```python
from build123d import *

# Parameters (mm, degrees)
BOSS_EXTRUDE1_DEPTH = 6
FILLET1_R           = 6
FILLET2_R           = 4
BOSS_EXTRUDE2_DEPTH = 12
LPATTERN1_COUNT     = 6
LPATTERN1_PITCH     = 6
CUT_EXTRUDE1_DEPTH  = 26
SKETCH5_R           = 1.5
CUT_EXTRUDE4_DEPTH  = 124.180869367
SKETCH6_R           = 1.75
BOSS_EXTRUDE3_DEPTH = 3
SKETCH7_R           = 1.25
CUT_EXTRUDE6_DEPTH  = 1
SKETCH8_R           = 1.25
CUT_EXTRUDE7_DEPTH  = 1
CUT_EXTRUDE8_DEPTH  = 1


with BuildPart() as part:
    # Sketch1 → Boss-Extrude1 (new, symmetric)
    with BuildSketch(Plane(origin=(0, 0, 0), x_dir=(1, 0, 0), z_dir=(0, 1, 0))):
        with BuildLine():
            ThreePointArc((13.432245527, -50.487906924), (21.509028276, -53.088979862), (18.907955338, -61.165762611))
            Line((18.907955338, -61.165762611), (11, -67.286566673))
            Line((11, -67.286566673), (11, -117.286566673))
            Line((11, -117.286566673), (0, -117.286566673))
            Line((0, -117.286566673), (0, -110.286566673))
            Line((0, -110.286566673), (-20.129396013, -88.042299634))
            Line((-20.129396013, -88.042299634), (-31.928362438, -82.58479184))
            Line((-31.928362438, -82.58479184), (-27.730279519, -73.508663821))
            Line((-27.730279519, -73.508663821), (-24.896421124, -73.027946621))
            Line((-24.896421124, -73.027946621), (-12.941547125, -71))
            Line((-12.941547125, -71), (-4.10711559, -69.126148868))
            Line((-4.10711559, -69.126148868), (13.432245527, -50.487906924))
        make_face()
        Polygon((-12.941547125, -71), (-24.896421124, -73.027946621), (-36.603518956, -4.013862114), (-12.941547125, 0), align=None)
    extrude(amount=BOSS_EXTRUDE1_DEPTH, both=True)

    # Fillet1
    fillet1_edges = [part.edges().sort_by_distance(p)[0] for p in [
        (-36.603518956, 0, 4.013862114),
        (-12.941547125, 0, 0),
    ]]
    fillet(fillet1_edges, radius=FILLET1_R)

    # Fillet2
    fillet2_edges = [part.edges().sort_by_distance(p)[0] for p in [
        (0, 0, 117.286566673),
        (-31.928362438, 0, 82.58479184),
        (-27.730279519, 0, 73.508663821),
    ]]
    fillet(fillet2_edges, radius=FILLET2_R)

    # Sketch2 → Boss-Extrude2 (add)
    with BuildSketch(Plane(origin=(0, 6, 0), x_dir=(1, 0, 0), z_dir=(0, 1, 0))):
        Polygon((15, -112.286566673), (11, -114.265571656), (11, -110.265571656), align=None)
    boss_extrude2 = extrude(amount=-BOSS_EXTRUDE2_DEPTH)

    # LPattern1: Boss-Extrude2 ×6
    with Locations(*[(0, 0, -i * LPATTERN1_PITCH) for i in range(1, LPATTERN1_COUNT)]):
        add(boss_extrude2)

    # Sketch3 → Cut-Extrude1 (cut)
    with BuildSketch(Plane(origin=(0, 6, 0), x_dir=(1, 0, 0), z_dir=(0, 1, 0))):
        Polygon((8.082911966, -112.457569416), (8.082911966, -87.457569416), (-6.917088034, -87.457569416), align=None)
    extrude(amount=-CUT_EXTRUDE1_DEPTH, mode=Mode.SUBTRACT)

    # Sketch5 → Cut-Extrude4 (cut, through all)
    with BuildSketch(Plane(origin=(0, 6, 0), x_dir=(1, 0, 0), z_dir=(0, 1, 0))):
        with Locations(Location((-29.68456047, -8.925889543, 0), (0, 0, 270))):
            Circle(SKETCH5_R)
    extrude(amount=-CUT_EXTRUDE4_DEPTH, mode=Mode.SUBTRACT)

    # Sketch6 → Boss-Extrude3 (add)
    with BuildSketch(Plane(origin=(0, 6, 0), x_dir=(1, 0, 0), z_dir=(0, 1, 0))):
        with Locations(Location((-26.618678063, -80.6335738, 0), (0, 0, 270))):
            Circle(SKETCH6_R)
        with Locations(Location((16.170100432, -55.826834767, 0), (0, 0, 270))):
            Circle(SKETCH6_R)
    boss_extrude3 = extrude(amount=BOSS_EXTRUDE3_DEPTH)

    # Sketch7 → Cut-Extrude6 (cut)
    with BuildSketch(Plane(origin=(0, 9, 0), x_dir=(1, 0, 0), z_dir=(0, 1, 0))):
        with Locations(Location((-26.618678063, -80.6335738, 0), (0, 0, 270))):
            Circle(SKETCH7_R)
    extrude(amount=-CUT_EXTRUDE6_DEPTH, mode=Mode.SUBTRACT)

    # Sketch8 → Cut-Extrude7 (cut)
    with BuildSketch(Plane(origin=(0, 9, 0), x_dir=(1, 0, 0), z_dir=(0, 1, 0))):
        with Locations(Location((16.170100432, -55.826834767, 0), (0, 0, 270))):
            Circle(SKETCH8_R)
    extrude(amount=-CUT_EXTRUDE7_DEPTH, mode=Mode.SUBTRACT)

    # Sketch9 → Cut-Extrude8 (cut)
    with BuildSketch(Plane(origin=(0, 6, 0), x_dir=(1, 0, 0), z_dir=(0, 1, 0))):
        with BuildLine():
            Line((-25.196199852, -15.539852581), (-16.757464085, -65.251677823))
            ThreePointArc((-16.757464085, -65.251677823), (-19.027845143, -68.450467492), (-22.226634811, -66.180086434))
            Line((-22.226634811, -66.180086434), (-30.665370577, -16.468261192))
            ThreePointArc((-30.665370577, -16.468261192), (-28.39498952, -13.269471524), (-25.196199852, -15.539852581))
        make_face()
    cut_extrude8 = extrude(amount=-CUT_EXTRUDE8_DEPTH, mode=Mode.SUBTRACT)

    # Mirror1: Boss-Extrude3, Cut-Extrude8 across plane
    add(boss_extrude3.mirror(Plane.ZX))
    add(cut_extrude8.mirror(Plane.ZX), mode=Mode.SUBTRACT)


solid = part.part
```
The listing builds one solid part. Answer for the finished solid, in the listing's coordinates (mm). A direction names the side the tool comes from. Give positions to 0.01 mm unless a question says otherwise; leave off trailing zeros. Loops run counter-clockwise (first coordinate to the right, second up) from the corner with the lowest first, then second, coordinate; pieces in that order, holes last. Notation, with made-up numbers: (-31.5, 22) - (-21.5, 22) arc R19 ccw to (-21.5, 30) - close; hole circle Ø3 at (-6.5, 87). An arc over 180 degrees is marked (long way). Return JSON: item names as keys, results as strings. Group by question number.
1. Find section B-B (z = 19). Write down the section's boundary in (x, y), then the cut area to 3 significant figures.
2. Find section D-D (z = 37.5). Write down the section's boundary in (x, y).
3. Find section C-C (y = 3). State how many separate pieces and enclosed holes the cut face has, then the cut area to 3 significant figures.
4. Determine the mould class of faces 1 (the cylindrical face through (-28.46, -5.51, 13.28)), 2 (the cylindrical face through (16.696, -7.479, 57.496)), 3 (the cylindrical face through (16.23, 8.51, 54.58)), 4 (the flat face through (13.03, 0.08, 113.26)) for opening direction X: pulls with the +X half, pulls with the -X half, needs draft (parallel to the pull), parting line crosses it, or undercut.
5. Straight lines are drawn through the part: line 1 (Z direction, x = -2, y = 0.75); line 2 (Y direction, x = 3, z = 105.5); line 3 (Z direction, x = -6.5, y = 0). For each, find the intervals that lie inside material, in ascending order. Write a range as [from, to].
6. Find section A-A (x = -5.5). Write down the section's boundary in (y, z).
7. Which of the six approach directions +Z, -Z, +X, -X, +Y, -Y give full straight-line access (tool end or side, diameter ignored) to faces 5 (the flat face through (13.03, 0.08, 107.26)), 6 (the flat face through (1, 0, 87.458)), 7 (the flat face through (-30.173, 0.084, 41.92))?
8. Given pin 1 Ø1.5 at (y, z) = (1.5, 111.5) entering from -X; pin 2 Ø1.6 at (y, z) = (2.5, 103.5) entering from +X; pin 3 Ø8 at (x, z) = (5.5, 91.5) entering from +Y; pin 4 Ø3 at (x, z) = (16.17, 55.83) entering from +Y, each flat-ended and moving along its own axis, determine where each tip first touches the part or whether it passes through.
Verdict:
{
 "1": {"outline": "(-34.06, -6) - (-30.24, -6) - (-30.24, -5) - (-24.61, -5) - (-24.61, -6) - (-12.94, -6) - (-12.94, 6) - (-24.61, 6) - (-24.61, 5) - (-30.24, 5) - (-30.24, 6) - (-34.06, 6) - close", "area": "242 mm^2"},
 "2": {"outline": "(-30.92, -6) - (-27.1, -6) - (-27.1, -5) - (-21.47, -5) - (-21.47, -6) - (-12.94, -6) - (-12.94, 6) - (-21.47, 6) - (-21.47, 5) - (-27.1, 5) - (-27.1, 6) - (-30.92, 6) - close"},
 "3": {"separate pieces": "1", "enclosed holes": "2", "area": "2,580 mm^2"},
 "4": {"face 1": "undercut", "face 2": "parting line crosses it", "face 3": "undercut", "face 4": "pulls with the +X half"},
 "5": {"line 1": "z = [66.89, 87.46], [95.65, 108.08]", "line 2": "y = [-6, 6]", "line 3": "z = [69.63, 87.46], [88.15, 103.1]"},
 "6": {"outline": "(-6, 69.42) - (6, 69.42) - (6, 87.46) - (-6, 87.46) - close; (-6, 89.82) - (6, 89.82) - (6, 104.21) - (-6, 104.21) - close"},
 "7": {"face 5": "+X, +Y, -Y", "face 6": "+Y, -Y", "face 7": "-X, +Y, -Y"},
 "8": {"pin 1": "stops at x = 0", "pin 2": "stops at x = 11.07", "pin 3": "stops at y = 6", "pin 4": "stops at y = 9"}
}
